Input: dimensioned drawing with shaded views. Units: mm. Origin: part minimum x, y, z. Round coordinates to 2 decimals unless told otherwise and drop trailing zeros. Loops run counter-clockwise (first coordinate to the right, second up) from the corner with the lowest first, then second, coordinate; pieces in that order, holes last. Notation, with made-up numbers: M 44.25,54.25 L 91.25,54.25 A11 ccw 91.25,59.25 Z; hole C -18.5,66.25 d6. An arc over 180 degrees is marked long. Write each question's results on one line, items separated by ' | '. Start each with the question number.
1. Section D-D on z = 2.25. Output: boundary loops of the cut face in (x, y).
2. Draft query along Y for the marked faces 1, 2 and 3. Return one class per face: released by +Y, released by -Y, zero draft, split by the parting line, or undercut.
3. Ray query, line 1 (Z direction, x = 19, y = 8.25); line 2 (X direction, y = 6, z = 12.5). Return the intervals inside material, ascending.
4. Section A-A on z = 9. Output: boundary loops of the cut face in (x, y), and give its area (3 significant figures).
5. Section B-B on x = 9. Output: boundary loops of the cut face in (y, z), and give its area (3 significant figures).
6. Section C-C on y = 12. Output: boundary loops of the cut face in (x, z).
7. Contact query for a flat-ended pin moving along its axis: pin 1 Ø3 at (y, z) = (9, 9) entering from -X. Output: stop coordinate, or through.
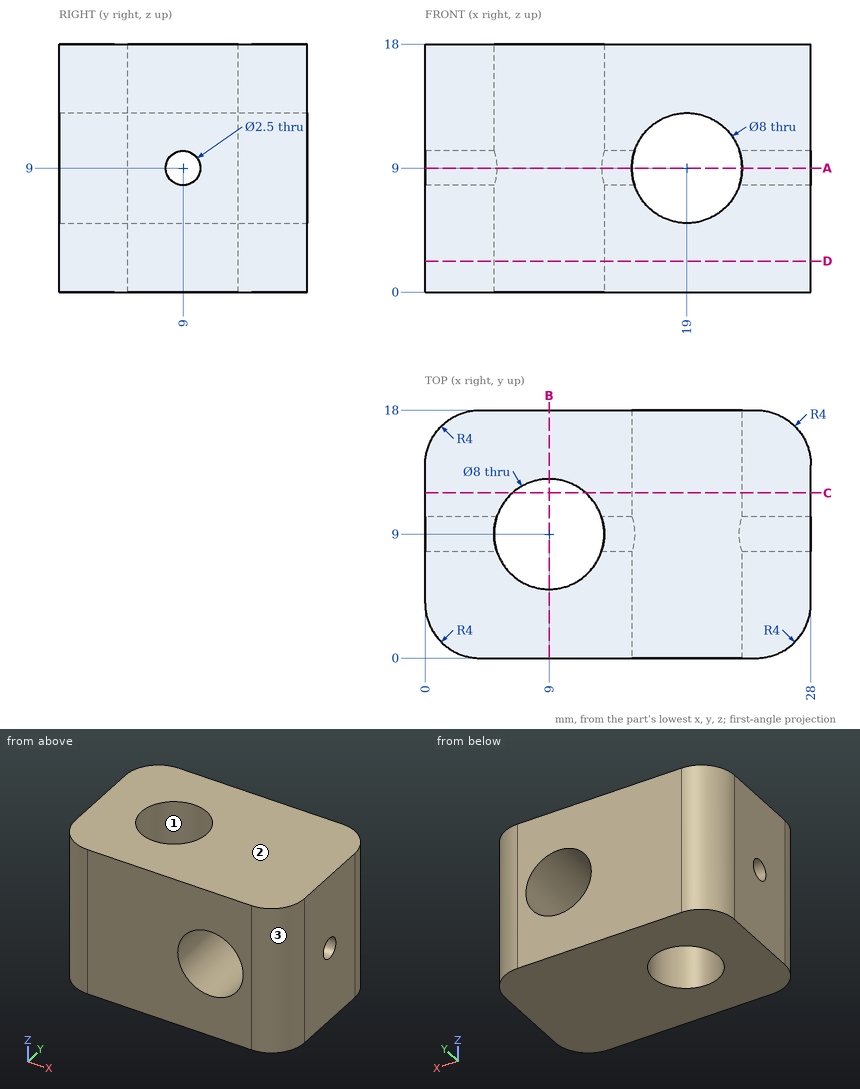
Taken from the geometry:
1) outline: M 0,4 A4 ccw 4,0 L 24,0 A4 ccw 28,4 L 28,14 A4 ccw 24,18 L 4,18 A4 ccw 0,14 Z; hole C 9,9 d8
2) face 1: undercut | face 2: zero draft | face 3: released by -Y
3) line 1: 0 to 5, 13 to 18 | line 2: 0 to 6.35, 11.65 to 17.06, 20.94 to 28
4) outline: M 0,4 A4 ccw 4,0 L 15,0 L 15,7.75 L 12.8,7.75 A4 cw 5.2,7.75 L 0,7.75 Z; M 0,10.25 L 5.2,10.25 A4 cw 12.8,10.25 L 15,10.25 L 15,18 L 4,18 A4 ccw 0,14 Z; M 23,0 L 24,0 A4 ccw 28,4 L 28,7.75 L 23,7.75 Z; M 23,10.25 L 28,10.25 L 28,14 A4 ccw 24,18 L 23,18 Z | area: 266 mm^2
5) outline: M 0,0 L 5,0 L 5,18 L 0,18 Z; M 13,0 L 18,0 L 18,18 L 13,18 Z | area: 180 mm^2
6) outline: M 0,0 L 6.35,0 L 6.35,18 L 0,18 Z; M 11.65,0 L 28,0 L 28,18 L 11.65,18 Z; hole C 19,9 d8
7) pin 1: x = 0
